from build123d import *

# Parameters (mm, degrees)
BOSS_EXTRU_1_DEPTH         = 4.07
BOSS_EXTRU_1_2_DEPTH       = 4.07
ESQUISSE1_3_W              = 15
ESQUISSE1_3_H              = 8
BOSS_EXTRU_2_DEPTH         = 32.04
BOSS_EXTRU_3_DEPTH         = 60.04
D_GAGEMENT_M31_D           = 3.2
D_GAGEMENT_M32_D           = 3.4
D_GAGEMENT_M32_DEPTH       = 6
D_GAGEMENT_START           = 22.75
D_GAGEMENT_M2_51_OUTLINE_R = 1.55
D_GAGEMENT_M2_51_DEPTH     = 8


# Read off the part's stored shape, not the designer's step: Dégagement M2.51
with BuildPart() as part:
    # Esquisse1 → Boss.-Extru.1 (new body)
    with BuildSketch(Plane.XY):
        Polygon((-52.5, -24.75), (-18.5, -24.75), (-18.5, -6.75), (-25.445395167, -6.75), (-25.445395167, 8.75), (-18.5, 8.75), (-18.5, 22.75), (-52.5, 22.75), align=None)
    extrude(amount=BOSS_EXTRU_1_DEPTH)



with BuildPart() as body_2:
    # Esquisse1 → Boss.-Extru.1 2 (new body)
    with BuildSketch(Plane.XY):
        Polygon((18.5, -24.75), (52.5, -24.75), (52.5, 22.75), (37.5, 22.75), (18.5, 22.75), (18.5, 8.75), (25.445395167, 8.75), (25.445395167, -6.75), (18.5, -6.75), align=None)
    extrude(amount=BOSS_EXTRU_1_2_DEPTH)


with BuildPart() as part_1:
    add(part.part)

    add(body_2.part)  # Boss.-Extru.2 merges body 2
    # Esquisse1<3> → Boss.-Extru.2 (add)
    with BuildSketch(Plane.XY):
        with Locations((-45, 26.75)):
            Rectangle(ESQUISSE1_3_W, ESQUISSE1_3_H)
        Polygon((-18.5, 8.75), (-18.5, -6.75), (-18.5, -24.75), (-52.5, -24.75), (-52.5, -30.75), (52.5, -30.75), (52.5, -24.75), (18.5, -24.75), (18.5, -6.75), (18.5, 8.75), (18.5, 22.75), (14.5, 22.75), (14.5, -28.75), (-14.5, -28.75), (-14.5, 22.75), (-18.5, 22.75), align=None)
        with Locations((45, 26.75)):
            Rectangle(ESQUISSE1_3_W, ESQUISSE1_3_H)
    extrude(amount=BOSS_EXTRU_2_DEPTH)

    # Esquisse1<4> → Boss.-Extru.3 (add)
    with BuildSketch(Plane.XY):
        Polygon((-37.5, 22.75), (-18.5, 22.75), (-14.5, 22.75), (14.5, 22.75), (18.5, 22.75), (37.5, 22.75), (37.5, 30.75), (-37.5, 30.75), align=None)
    extrude(amount=BOSS_EXTRU_3_DEPTH)

    # Dégagement M31 (through all)
    with Locations(Plane.ZY.offset(18.5)):
        with Locations((8.07, -21), (8.07, 19), (30.07, 19), (30.07, -21)):
            Hole(D_GAGEMENT_M31_D / 2)

    # Dégagement M32
    with Locations(Plane(origin=(0, -30.75, 0), x_dir=(-1, 0, 0), z_dir=(0, -1, 0))):
        with Locations((-41.5, -25.52), (-41.5, -6.52), (41.5, -6.52), (41.5, -25.52)):
            Hole(D_GAGEMENT_M32_D / 2, depth=D_GAGEMENT_M32_DEPTH)

    # Dégagement M2.51 outline → Dégagement M2.51 (cut)
    with BuildSketch(Plane(origin=(0, 0, 0), x_dir=(1, 0, 0), z_dir=(0, 1, 0)).offset(D_GAGEMENT_START)):
        with Locations((0, -54.04)):
            Circle(D_GAGEMENT_M2_51_OUTLINE_R)
        with Locations((0, -25.04)):
            Circle(D_GAGEMENT_M2_51_OUTLINE_R)
    extrude(amount=D_GAGEMENT_M2_51_DEPTH, mode=Mode.SUBTRACT)


solid = part_1.part
Geometry: final body of the model. Coordinates: model frame, mm. A direction names the side the tool comes from. Give positions to 0.01 mm unless a question says otherwise; leave off trailing zeros. Order: outer loops, then holes, each group sorted by start corner. A loop starts at its lowest first (then second) coordinate and runs counter-clockwise, first axis right, second up. Notation, with made-up numbers: (38.25, 29) -> (96.25, 29) arc R13 cw to (96.25, 41) -> close; hole circle Ø3 at (-1.75, 86.25). An arc over 180 degrees is marked (long way). Put each result on its own line as item: value.
Q1. Section B-B, the plane y = 19. Return loops of the section in (x, z).
Here are the results:
outline: (-52.5, 0) -> (-14.5, 0) -> (-14.5, 6.47) -> (-18.5, 6.47) -> (-18.5, 4.07) -> (-52.5, 4.07) -> close; (-18.5, 9.67) -> (-14.5, 9.67) -> (-14.5, 28.47) -> (-18.5, 28.47) -> close; (-18.5, 31.67) -> (-14.5, 31.67) -> (-14.5, 32.04) -> (-18.5, 32.04) -> close; (14.5, 0) -> (52.5, 0) -> (52.5, 4.07) -> (18.5, 4.07) -> (18.5, 6.47) -> (14.5, 6.47) -> close; (14.5, 9.67) -> (18.5, 9.67) -> (18.5, 28.47) -> (14.5, 28.47) -> close; (14.5, 31.67) -> (18.5, 31.67) -> (18.5, 32.04) -> (14.5, 32.04) -> close
Q2. Reachability of faces 1 (the face through (45, 27, 32.04)), 2 (the face through (-1, 22.75, 30)), 3 (the face through (-42.75, -27.71, 5.37)), 4 (the face through (35, -1, 4.07)) from +Z, -Z, +X, -X, +Y, -Y: full face, straight path, thin tool, end or side. Return the list, or none.
Here are the results:
face 1: +Z, +X, +Y, -Y
face 2: +Z
face 3: -Y
face 4: +Z, +X
Q3. Draft query along X for faces 5 (the face through (22, -6.75, 2)), 6 (the face through (0.715, 26.694, 26.415)), 7 (the face through (36, -24.75, 18)), 8 (the face through (-52.5, -2, 3)). Return one class per face: released by +X, released by -X, zero draft, split by the parting line, or undercut.
Here are the results:
face 5: undercut
face 6: undercut
face 7: zero draft
face 8: released by -X
Q4. Material intervals for L1, parallel to Y at x = 17, z = 8; L2, parallel to X at y = -29, z = 25.52; L3, parallel to Y at x = -43.5, z = 17, sorted ascending.
Here are the results:
L1: y = -30.75 to -22.6, -19.4 to 17.4, 20.6 to 30.75
L2: x = -52.5 to -43.2, -39.8 to 39.8, 43.2 to 52.5
L3: y = -30.75 to -24.75, 22.75 to 30.75
Q5. Section A-A, the plane x = 41.5. Return loops of the section in (y, z).
Here are the results:
outline: (-30.75, 0) -> (30.75, 0) -> (30.75, 32.04) -> (22.75, 32.04) -> (22.75, 4.07) -> (-24.75, 4.07) -> (-24.75, 4.82) -> (-30.75, 4.82) -> close; (-30.75, 8.22) -> (-24.75, 8.22) -> (-24.75, 23.82) -> (-30.75, 23.82) -> close; (-30.75, 27.22) -> (-24.75, 27.22) -> (-24.75, 32.04) -> (-30.75, 32.04) -> close
Q6. Section C-C, the plane x = 12. Return loops of the section in (y, z).
Here are the results:
outline: (-30.75, 0) -> (-28.75, 0) -> (-28.75, 32.04) -> (-30.75, 32.04) -> close; (22.75, 0) -> (30.75, 0) -> (30.75, 60.04) -> (22.75, 60.04) -> close
Q7. Section D-D, the plane z = 30.07. Count the separate pieces of the cut face and the enclosed holes in it, then the cut area to 3 significant figures.
Here are the results:
separate pieces: 4
enclosed holes: 0
area: 1,680 mm^2
Q8. Pin query (flat end, axial travel): pin 1 (3.5 mm diameter, centred on y = -21, z = 30.07, fed in from -X); pin 2 (1.9 mm diameter, centred on y = 19, z = 8.07, fed in from +X); pin 3 (9 mm diameter, centred on x = 48.5, y = 26, fed in from +Z); pin 4 (1.5 mm diameter, centred on x = -26, y = -23.5, fed in from +Z). Return the tip coordinate at first contact, or that it passes through.
Here are the results:
pin 1: stops at x = -18.5
pin 2: passes through
pin 3: stops at z = 32.04
pin 4: stops at z = 4.07
